Input: dimensioned drawing with shaded views. Units: mm. Origin: part minimum x, y, z. A direction names the side the tool comes from. Give positions to 0.01 mm unless a question says otherwise; leave off trailing zeros. Write each loop counter-clockwise with the first axis right and the second up, starting at its lowest first coordinate (ties: lowest second). Pieces come first, ordered by that corner, then holes.
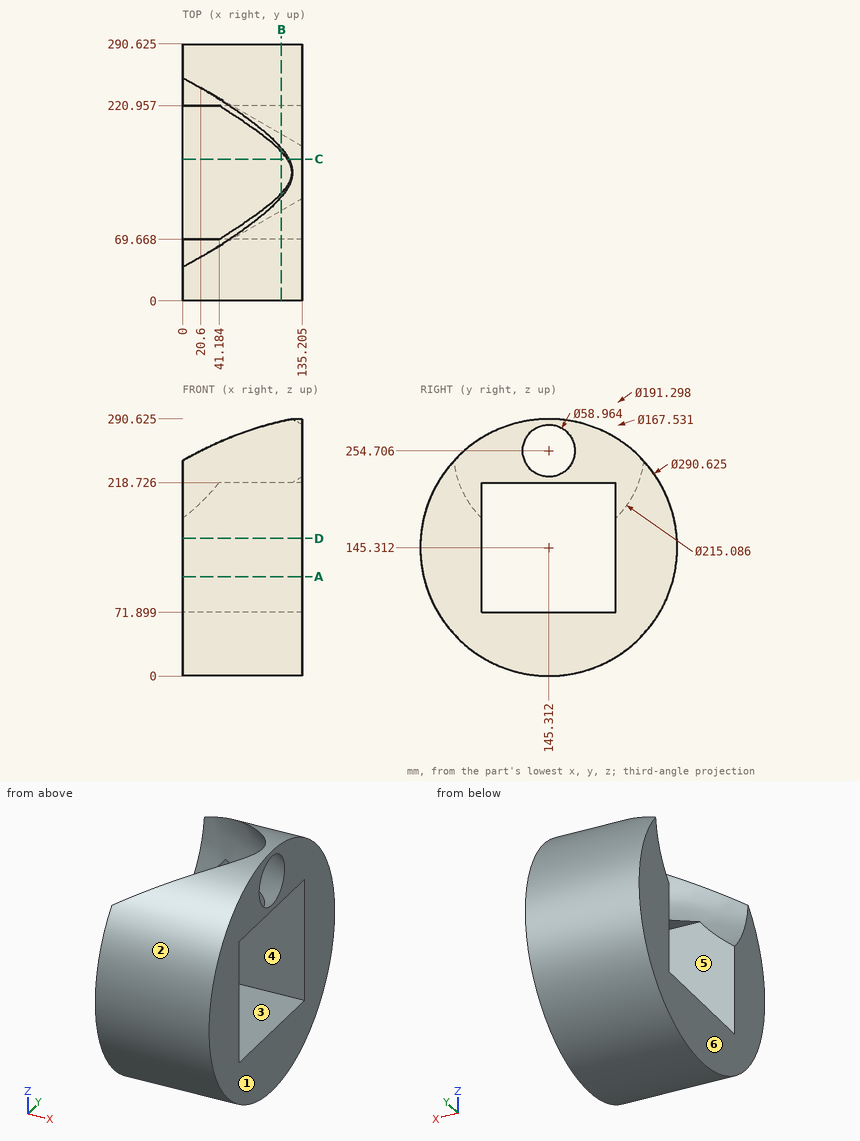
Item 1: Pin query (flat end, axial travel): pin 1 Ø6 at (x, z) = (36.5, 221.5) entering from -Y; pin 2 Ø1 at (x, y) = (17, 261) entering from +Z; pin 3 Ø3 at (x, y) = (120, 151.5) entering from +Z. Return the tip coordinate at first contact, or that it passes through.
Found:
pin 1: stops at y = 19.78
pin 2: stops at z = 233.9
pin 3: stops at z = 71.9
Item 2: Section D-D, the plane z = 155.5. Return the cut outline in (x, y) (1 decimal).
Found:
outline: (0, 0.4) - (135.2, 0.4) - (135.2, 69.7) - (0, 69.7) - close; (0, 221) - (135.2, 221) - (135.2, 290.3) - (0, 290.3) - close
Item 3: Line query: L1, parallel to Y at x = 102.5, z = 144 (1 decimal); L2, parallel to Y at x = 125, z = 90 (1 decimal); L3, parallel to Z at x = 21, y = 140. Output: solid intervals per line, ascending.
Found:
L1: y = 0 to 69.7, 221 to 290.6
L2: y = 10.9 to 69.7, 221 to 279.7
L3: z = 0.1 to 71.9
Item 4: Pull-direction query (Y, two-part tool) for the marked faces 1, 2, 3 and 4; classes: +Y half, -Y half, draft (parallel to the pull), parting line (faces both ways), or undercut.
Found:
face 1: draft
face 2: parting line
face 3: undercut
face 4: undercut
Item 5: Section B-B, the plane x = 111.5. Return the cut outline in (y, z) (1 decimal), plus the area to 3 significant figures.
Found:
outline: (69.7, 71.9) - (69.7, 218.7) - (121.5, 218.7) arc R43.2 cw to (117.8, 288) arc R145.3 ccw (long way) to (172.8, 288) arc R43.2 cw to (169.2, 218.7) - (221, 218.7) - (221, 71.9) - close
area: 38,800 mm2
Item 6: Reachability of the marked faces 5 and 6 from +Z, -Z, +X, -X, +Y, -Y: full face, straight path, thin tool, end or side. Return the list, or none.
Found:
face 5: +X, -X
face 6: +Z, -Z, -X, +Y, -Y
Item 7: Section A-A, the plane z = 112.5. Return the cut outline in (x, y) (1 decimal).
Found:
outline: (0, 3.8) - (135.2, 3.8) - (135.2, 69.7) - (0, 69.7) - close; (0, 221) - (135.2, 221) - (135.2, 286.9) - (0, 286.9) - close
Item 8: Section C-C, the plane y = 160.5. State how many separate pieces and enclosed holes the cut face has.
Found:
separate pieces: 3
enclosed holes: 0
